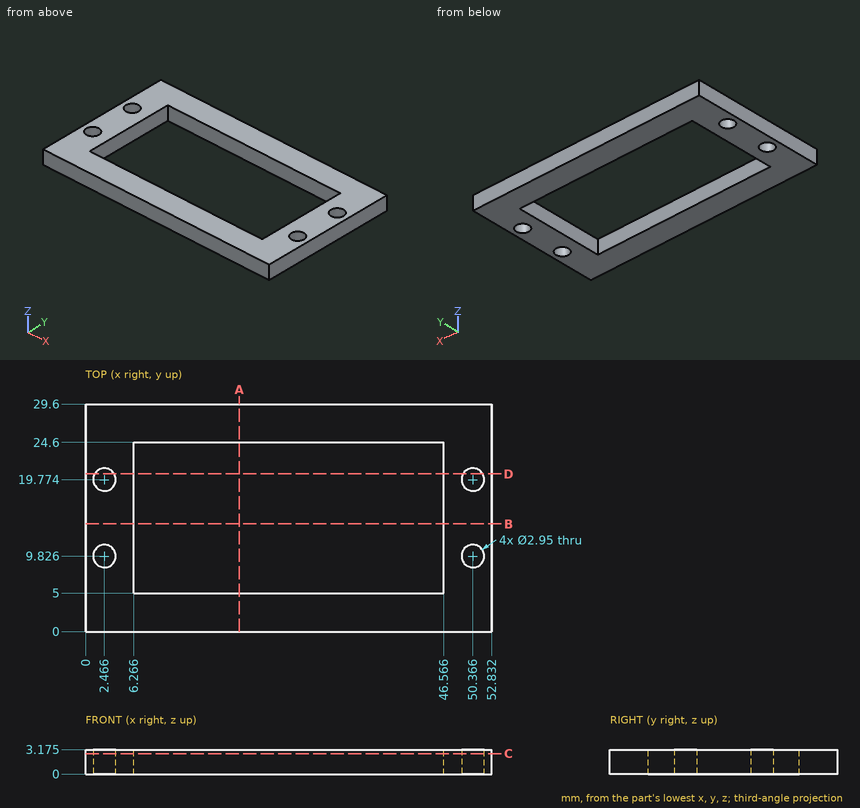
Study the drawing (mm; zero at the part's minimum x, y, z) and answer. Round coordinates to 2 decimals unless told otherwise and drop trailing zeros. Loops run counter-clockwise (first coordinate to the right, second up) from the corner with the lowest first, then second, coordinate; pieces in that order, holes last.
Q1. Section C-C, the plane z = 2.65 is taken. Determine the outline of the cut face in (x, y) (3 decimals), then the cut area to 3 significant figures.
Q2. Section A-A, the plane x = 20 is taken. Determine the outline of the cut face in (y, z) (3 decimals), then the cut area to 4 significant figures.
Q3. Section B-B, the plane y = 14 is taken. Determine the outline of the cut face in (x, z) (3 decimals).
Q4. Section D-D, the plane y = 20.5 is taken. Determine the outline of the cut face in (x, z) (3 decimals).
Q5. Find the intervals of material crossed by line 1 (Y direction, x = 22.5, z = 0.45); line 2 (X direction, y = 5.75, z = 2.4); line 3 (X direction, y = 8.5, z = 0.85), in increasing order.
Completed:
1. outline: (0, 0) - (52.832, 0) - (52.832, 29.6) - (0, 29.6) - close; hole circle Ø2.95 at (2.466, 9.826); hole circle Ø2.95 at (2.466, 19.774); hole (6.266, 5) - (46.566, 5) - (46.566, 24.6) - (6.266, 24.6) - close; hole circle Ø2.95 at (50.366, 9.826); hole circle Ø2.95 at (50.366, 19.774)
1. area: 747 mm2
2. outline: (0, 0) - (5, 0) - (5, 3.175) - (0, 3.175) - close; (24.6, 0) - (29.6, 0) - (29.6, 3.175) - (24.6, 3.175) - close
2. area: 31.75 mm2
3. outline: (0, 0) - (6.266, 0) - (6.266, 3.175) - (0, 3.175) - close; (46.566, 0) - (52.832, 0) - (52.832, 3.175) - (46.566, 3.175) - close
4. outline: (0, 0) - (1.182, 0) - (1.182, 3.175) - (0, 3.175) - close; (3.75, 0) - (6.266, 0) - (6.266, 3.175) - (3.75, 3.175) - close; (46.566, 0) - (49.082, 0) - (49.082, 3.175) - (46.566, 3.175) - close; (51.65, 0) - (52.832, 0) - (52.832, 3.175) - (51.65, 3.175) - close
5. line 1: y = 0 to 5, 24.6 to 29.6
5. line 2: x = 0 to 6.27, 46.57 to 52.83
5. line 3: x = 0 to 1.82, 3.11 to 6.27, 46.57 to 49.72, 51.01 to 52.83
